Autodesk Inventor part; units mm, degrees
ref_plane "YZ Plane" through (0, 0, 0) normal (1, 0, 0) x (0, 1, 0)
ref_plane "XZ Plane" through (0, 0, 0) normal (0, 1, 0) x (-1, 0, 0)
ref_plane "XY Plane" through (0, 0, 0) normal (0, 0, 1) x (1, 0, 0)
ref_plane "Work Plane1" through (0, 0, 0) normal (0, 0, 1) x (1, 0, 0)
sketch "Sketch1" plane through (0, 0, 0) normal (0, 0, 1) x (1, 0, 0)
  line L0 (25.2394, 234.4042) -> (-62.7606, 234.4042)
  line L1 (-62.7606, 234.4042) -> (-62.7606, 144.9042)
  line L2 (-62.7606, 144.9042) -> (25.2394, 144.9042)
  line L3 (25.2394, 144.9042) -> (25.2394, 234.4042)
  line L4 (23.4394, 232.6042) -> (-60.9606, 232.6042)
  line L5 (-60.9606, 232.6042) -> (-60.9606, 146.7042)
  line L6 (-60.9606, 146.7042) -> (23.4394, 146.7042)
  line L7 (23.4394, 146.7042) -> (23.4394, 232.6042)
  circle A0 centre (21.9394, 231.1042) radius 3.3
  circle A1 centre (21.9394, 231.1042) radius 1.5
  line L8 (-18.7606, 249.1641) -> (-18.7606, 136.0401)
  line L9 (-67.3062, 189.6542) -> (41.0259, 189.6542)
  circle A2 centre (-59.4606, 231.1042) radius 3.3
  circle A3 centre (-59.4606, 231.1042) radius 1.5
  circle A4 centre (21.9394, 148.2042) radius 3.3
  circle A5 centre (21.9394, 148.2042) radius 1.5
  circle A6 centre (-59.4606, 148.2042) radius 3.3
  circle A7 centre (-59.4606, 148.2042) radius 1.5
  line L10 (2.7394, 221.1042) -> (16.7394, 221.1042)
  line L11 (16.7394, 221.1042) -> (16.7394, 207.1042)
  line L12 (16.7394, 207.1042) -> (2.7394, 207.1042)
  line L13 (2.7394, 207.1042) -> (2.7394, 221.1042)
  line L14 (-16.2606, 221.1042) -> (-2.2606, 221.1042)
  line L15 (-2.2606, 221.1042) -> (-2.2606, 207.1042)
  line L16 (-2.2606, 207.1042) -> (-16.2606, 207.1042)
  line L17 (-16.2606, 207.1042) -> (-16.2606, 221.1042)
  line L18 (2.7394, 202.1042) -> (16.7394, 202.1042)
  line L19 (16.7394, 202.1042) -> (16.7394, 188.1042)
  line L20 (16.7394, 188.1042) -> (2.7394, 188.1042)
  line L21 (2.7394, 188.1042) -> (2.7394, 202.1042)
  line L22 (-16.2606, 202.1042) -> (-2.2606, 202.1042)
  line L23 (-2.2606, 202.1042) -> (-2.2606, 188.1042)
  line L24 (-2.2606, 188.1042) -> (-16.2606, 188.1042)
  line L25 (-16.2606, 188.1042) -> (-16.2606, 202.1042)
  line L26 (2.7394, 183.1042) -> (16.7394, 183.1042)
  line L27 (16.7394, 183.1042) -> (16.7394, 169.1042)
  line L28 (16.7394, 169.1042) -> (2.7394, 169.1042)
  line L29 (2.7394, 169.1042) -> (2.7394, 183.1042)
  line L30 (-2.2606, 169.1042) -> (-16.2606, 169.1042)
  line L31 (-16.2606, 169.1042) -> (-16.2606, 183.1042)
  line L32 (-16.2606, 183.1042) -> (-2.2606, 183.1042)
  line L33 (-2.2606, 183.1042) -> (-2.2606, 169.1042)
  line L34 (16.7394, 150.1042) -> (2.7394, 150.1042)
  line L35 (2.7394, 150.1042) -> (2.7394, 164.1042)
  line L36 (2.7394, 164.1042) -> (16.7394, 164.1042)
  line L37 (16.7394, 164.1042) -> (16.7394, 150.1042)
  line L38 (-2.2606, 150.1042) -> (-16.2606, 150.1042)
  line L39 (-16.2606, 150.1042) -> (-16.2606, 164.1042)
  line L40 (-16.2606, 164.1042) -> (-2.2606, 164.1042)
  line L41 (-2.2606, 164.1042) -> (-2.2606, 150.1042)
  line L42 (-35.2606, 221.1042) -> (-21.2606, 221.1042)
  line L43 (-21.2606, 221.1042) -> (-21.2606, 207.1042)
  line L44 (-21.2606, 207.1042) -> (-35.2606, 207.1042)
  line L45 (-35.2606, 207.1042) -> (-35.2606, 221.1042)
  line L46 (-40.2606, 207.1042) -> (-54.2606, 207.1042)
  line L47 (-54.2606, 207.1042) -> (-54.2606, 221.1042)
  line L48 (-54.2606, 221.1042) -> (-40.2606, 221.1042)
  line L49 (-40.2606, 221.1042) -> (-40.2606, 207.1042)
  line L50 (-21.2606, 188.1042) -> (-35.2606, 188.1042)
  line L51 (-35.2606, 188.1042) -> (-35.2606, 202.1042)
  line L52 (-35.2606, 202.1042) -> (-21.2606, 202.1042)
  line L53 (-21.2606, 202.1042) -> (-21.2606, 188.1042)
  line L54 (-40.2606, 188.1042) -> (-54.2606, 188.1042)
  line L55 (-54.2606, 188.1042) -> (-54.2606, 202.1042)
  line L56 (-54.2606, 202.1042) -> (-40.2606, 202.1042)
  line L57 (-40.2606, 202.1042) -> (-40.2606, 188.1042)
  line L58 (-40.2606, 150.1042) -> (-54.2606, 150.1042)
  line L59 (-54.2606, 164.1042) -> (-40.2606, 164.1042)
  line L60 (-54.2606, 150.1042) -> (-54.2606, 164.1042)
  line L61 (-40.2606, 164.1042) -> (-40.2606, 150.1042)
  line L62 (-35.2606, 150.1042) -> (-35.2606, 164.1042)
  line L63 (-35.2606, 164.1042) -> (-21.2606, 164.1042)
  line L64 (-21.2606, 150.1042) -> (-35.2606, 150.1042)
  line L65 (-21.2606, 164.1042) -> (-21.2606, 150.1042)
  line L66 (-21.2606, 169.1042) -> (-35.2606, 169.1042)
  line L67 (-40.2606, 169.1042) -> (-54.2606, 169.1042)
  line L68 (-35.2606, 183.1042) -> (-21.2606, 183.1042)
  line L69 (-21.2606, 183.1042) -> (-21.2606, 169.1042)
  line L70 (-35.2606, 169.1042) -> (-35.2606, 183.1042)
  line L71 (-40.2606, 183.1042) -> (-40.2606, 169.1042)
  line L72 (-54.2606, 183.1042) -> (-40.2606, 183.1042)
  line L73 (-54.2606, 169.1042) -> (-54.2606, 183.1042)
  point P0 (-18.7606, 189.6542)
  point P1 (-18.7606, 234.4042)
  point P2 (-18.7606, 189.6542)
  point P3 (25.2394, 189.6542)
  dimension "d0" = 88
  dimension "d1" = 89.5
  dimension "d2" = 84.4
  dimension "d3" = 85.9
  dimension "d4" = 1.8
  dimension "d5" = 1.8
  dimension "d6" = 6.6
  dimension "d7" = 3.3
  dimension "d8" = 3.3
  dimension "d9" = 3
  dimension "d12" = 44.75
  dimension "d13" = 44
  dimension "d70" = 84.4
  dimension "d71" = 85.9
  dimension "d81" = 14
  dimension "d82" = 14
  dimension "d83" = 14
  dimension "d84" = 14
  dimension "d85" = 5
  dimension "d86" = 14
  dimension "d87" = 14
  dimension "d88" = 5
  dimension "d89" = 14
  dimension "d90" = 14
  dimension "d91" = 5
  dimension "d92" = 5
  dimension "d93" = 14
  dimension "d94" = 14
  dimension "d95" = 14
  dimension "d96" = 14
  dimension "d97" = 5
  dimension "d98" = 14
  dimension "d99" = 14
  dimension "d100" = 5
  dimension "d101" = 14
  dimension "d102" = 14
  dimension "d103" = 5
  dimension "d104" = 5
  dimension "d105" = 5
  dimension "d106" = 5
  dimension "d107" = 11.5
  dimension "d108" = 11.5
  dimension "d109" = 14
  dimension "d110" = 14
  dimension "d111" = 14
  dimension "d112" = 14
  dimension "d113" = 5
  dimension "d114" = 14
  dimension "d115" = 14
  dimension "d116" = 5
  dimension "d117" = 14
  dimension "d118" = 14
  dimension "d119" = 5
  dimension "d120" = 5
  dimension "d121" = 14
  dimension "d122" = 14
  dimension "d123" = 14
  dimension "d124" = 14
  dimension "d125" = 5
  dimension "d126" = 14
  dimension "d127" = 14
  dimension "d128" = 5
  dimension "d129" = 14
  dimension "d130" = 14
extrude "Extrusion2" add sketch "Sketch1" against normal blind 1.8 contours L3 A0 L0 | A0 L4 L8 L0 | A0 L7 L4 | L3 L9 L7 A0 | A0 L7 L9 L19 L18 L21 L23 L22 L25 L8 L4 | L4 A1 L7 A0 | L4 L7 A1 | L9 L21 L18 L19 | L25 L22 L23 L9 | L10 L11 L12 L13 | L14 L15 L16 L17
hole "Hole2" at (21.9394, 231.1042, 0) direction (0, 0, -1) diameter 3 end through all countersink diameter 6 countersink angle 80
ref_plane "Work Plane4" through (-18.7606, 189.6542, -1.8) normal (1, 0, 0) x (0, 1, 0)
ref_plane "Work Plane5" through (-18.7606, 189.6542, 0) normal (0, -1, 0) x (1, 0, 0)
fillet "Fillet3" radius 3 1 edges at (25.2394, 234.4042, -0.9)
mirror "Mirror5" about plane through (-18.7606, 189.6542, 0) normal (0, -1, 0)
mirror "Mirror6" about plane through (-18.7606, 189.6542, -1.8) normal (1, 0, 0)
extrude "Extrusion3" cut sketch "Sketch1" against normal blind 1.5 contours L19 L20 L21 L9 | L9 L21 L18 L19 | L53 L50 L51 L9 | L9 L51 L52 L53 | L25 L22 L23 L9 | L9 L23 L24 L25 | L55 L56 L57 L9 | L9 L57 L54 L55 | L10 L11 L12 L13 | L14 L15 L16 L17 | L26 L27 L28 L29 | L30 L31 L32 L33 | L34 L35 L36 L37 | L38 L39 L40 L41 | L42 L43 L44 L45 | L46 L47 L48 L49 | L58 L60 L59 L61 | L62 L63 L65 L64 | L66 L70 L68 L69 | L67 L73 L72 L71
equation "\"d2\" = d0 - 2 * d4"
equation "\"d3\" = d1 - 2 * d5"
equation "\"d5\" = d4"
equation "\"d6\" = 2 * d4 + d9"
equation "\"d7\" = 0.5 * d6"
equation "\"d8\" = 0.5 * d6"
properties part number "plate"
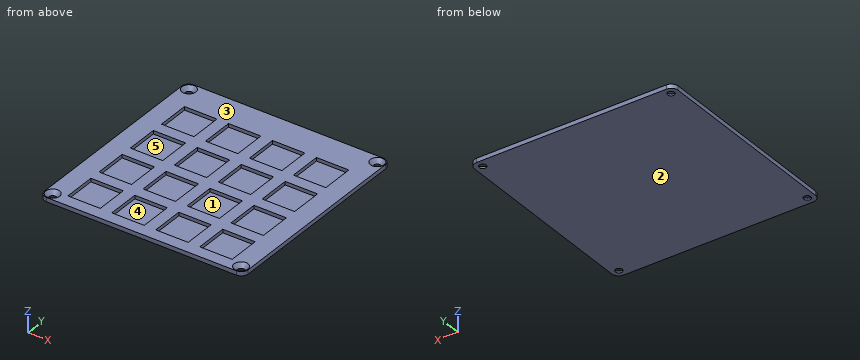
The listing builds one solid part. Answer for the finished solid, in the listing's coordinates (mm). Face numbers are marked on the shaded views. A direction names the side the tool comes from. Round coordinates to 2 decimals unless told otherwise and drop trailing zeros. Order: outer loops, then holes, each group sorted by start corner. A loop starts at its lowest first (then second) coordinate and runs counter-clockwise, first axis right, second up. Notation, with made-up numbers: (77.25, 68.5) -> (116.25, 68.5) arc R20 ccw to (116.25, 85.5) -> close; hole circle Ø3 at (18, -11.5). An arc over 180 degrees is marked (long way). Put each result on its own line as item: value.
Q1. Determine the mould class of the marked faces 3, 4 and 5 for opening direction X: pulls with the +X half, pulls with the -X half, needs draft (parallel to the pull), parting line crosses it, or undercut.
Results list:
face 3: needs draft
face 4: undercut
face 5: undercut
Q2. Section A-A, the plane x = -46.5 is taken. Write down the section's boundary in (y, z).
Results list:
outline: (144.9, -1.8) -> (234.4, -1.8) -> (234.4, 0) -> (221.1, 0) -> (221.1, -1.5) -> (207.1, -1.5) -> (207.1, 0) -> (202.1, 0) -> (202.1, -1.5) -> (188.1, -1.5) -> (188.1, 0) -> (183.1, 0) -> (183.1, -1.5) -> (169.1, -1.5) -> (169.1, 0) -> (164.1, 0) -> (164.1, -1.5) -> (150.1, -1.5) -> (150.1, 0) -> (144.9, 0) -> close
Q3. Section C-C, the plane z = -0.65 is taken. Count the separate pieces of the cut face and the enclosed holes in it, and give its area (3 significant figures).
Results list:
separate pieces: 1
enclosed holes: 20
area: 4,660 mm^2
Q4. Consider line 1 along Y through (x, z) = (-49, -1.3); line 2 along X through (y, z) = (177.5, -0.2); line 3 along Y through (x, z) = (-59, -0.2). Determine where each line is inside the solid, lowest interval first.
Results list:
line 1: 144.9 to 150.1, 164.1 to 169.1, 183.1 to 188.1, 202.1 to 207.1, 221.1 to 234.4
line 2: -62.76 to -54.26, -40.26 to -35.26, -21.26 to -16.26, -2.26 to 2.74, 16.74 to 25.24
line 3: 144.9 to 145.41, 151 to 228.31, 233.9 to 234.4
Q5. Section B-B, the plane y = 217 is taken. Write down the section's boundary in (x, z).
Results list:
outline: (-62.76, -1.8) -> (25.24, -1.8) -> (25.24, 0) -> (16.74, 0) -> (16.74, -1.5) -> (2.74, -1.5) -> (2.74, 0) -> (-2.26, 0) -> (-2.26, -1.5) -> (-16.26, -1.5) -> (-16.26, 0) -> (-21.26, 0) -> (-21.26, -1.5) -> (-35.26, -1.5) -> (-35.26, 0) -> (-40.26, 0) -> (-40.26, -1.5) -> (-54.26, -1.5) -> (-54.26, 0) -> (-62.76, 0) -> close
Q6. Which of the six approach directions +Z, -Z, +X, -X, +Y, -Y give full straight-line access (tool end or side, diameter ignored) to the marked faces 1 and 2?
Results list:
face 1: +Z
face 2: -Z, +X, -X, +Y, -Y
Q7. Each of these flat-tipped pins is pushed along its axis until it touches: P1, Ø5, axis at x = 21.94, y = 231.1, coming from the +Z side; P2, Ø15.5, axis at x = -45.5, y = 154.5, coming from the +Z side; P3, Ø4, axis at x = -6, y = 195.5, coming from the +Z side. Where does it stop, or does it pass through?
Results list:
P1: z = -0.59
P2: z = 0
P3: z = -1.5
